The model under review builds one solid part; all positions refer to its coordinate system, in mm. A direction names the side the tool comes from. Give positions to 0.01 mm unless a question says otherwise; leave off trailing zeros. Write each loop counter-clockwise with the first axis right and the second up, starting at its lowest first coordinate (ties: lowest second). Pieces come first, ordered by that corner, then holes.
from build123d import *

# Parameters (mm, degrees)
SKETCH_1_W          = 15
SKETCH_1_H          = 15
SKETCH_1_W_2        = 12
SKETCH_1_H_2        = 12
EXTRUDE_2_DEPTH     = 30
SKETCH_2_R          = 1
CUT_EXTRUDE_1_DEPTH = 10
SKETCH_3_R          = 1.5
CUT_EXTRUDE_2_DEPTH = 10
SKETCH_5_R          = 1.5
CUT_EXTRUDE_4_DEPTH = 10


with BuildPart() as part:
    # ｽｹｯﾁ1 → ﾎﾞｽ - 押し出し2 (new body)
    with BuildSketch(Plane.XY):
        with Locations((0.489915859, 0.232626086)):
            Rectangle(SKETCH_1_W, SKETCH_1_H)
        with Locations((0.489915859, 0.232626086)):
            Rectangle(SKETCH_1_W_2, SKETCH_1_H_2, mode=Mode.SUBTRACT)
    extrude(amount=EXTRUDE_2_DEPTH)

    # ｽｹｯﾁ2 → ｶｯﾄ - 押し出し1 (cut)
    with BuildSketch(Plane(origin=(0, 7.732626086, 0), x_dir=(1, 0, 0), z_dir=(0, 1, 0))):
        with Locations((3.689915859, -25.6)):
            Circle(SKETCH_2_R)
        with Locations((3.689915859, -14.8)):
            Circle(SKETCH_2_R)
    extrude(amount=-CUT_EXTRUDE_1_DEPTH, mode=Mode.SUBTRACT)

    # ｽｹｯﾁ3 → ｶｯﾄ - 押し出し2 (cut)
    with BuildSketch(Plane.ZY.offset(7.010084141)):
        with Locations((7.5, 0.232626086)):
            Circle(SKETCH_3_R)
    extrude(amount=-CUT_EXTRUDE_2_DEPTH, mode=Mode.SUBTRACT)

    # ｽｹｯﾁ5 → ｶｯﾄ - 押し出し4 (cut)
    with BuildSketch(Plane.XZ.offset(7.267373914)):
        with Locations((0.489915859, 22.5)):
            Circle(SKETCH_5_R)
    extrude(amount=-CUT_EXTRUDE_4_DEPTH, mode=Mode.SUBTRACT)


solid = part.part
1) Consider section D-D, the plane x = 3. Give the boundary of the cut face in (y, z).
2) To check wall thickness, follow probe 1 along X at (y, z) = (-2.5, 14.75); probe 2 along Y at (x, z) = (5.25, 24.25); probe 3 along Y at (x, z) = (-6.05, 7.5). State the ranges of each line that lie inside material, in increasing order.
3) Consider section C-C, the plane z = 14.8. Give the boundary of the cut face in (x, y), then the cut area to 3 significant figures.
4) Consider section A-A, the plane x = -1.75. Give the boundary of the cut face in (y, z), then the cut area to 3 significant figures.
5) Insertion check: pin 1 (2.5 mm diameter, centred on x = 0.49, z = 22.5, fed in from -Y). The pin has a flat end and moves straight along its axis. Give the tip position at first contact, or say it passes through.
6) Consider section B-B, the plane y = 5.75. Give the boundary of the cut face in (x, z).
7) Tool access review of faces 4 (the cylindrical face through (-6.27, -0.68, 6.31)), 5 (the cylindrical face through (4.15, 6.99, 15.69)), 6 (the flat face through (-5.51, 0, 15)): name each direction out of +Z, -Z, +X, -X, +Y, -Y from which nothing blocks a thin tool from reaching the whole face with its end or side.
8) The part is to be moulded in two halves that separate along Z. For faces 1 (the flat face through (-6, 0, 0)), 2 (the flat face through (0, -7.267, 15)), 3 (the cylindrical face through (3.56, 6.99, 24.61)), say which applies: +Z half, -Z half, draft (parallel to the pull), parting line (faces both ways), or undercut.
Answer block:
1. outline: (-7.27, 0) - (-5.77, 0) - (-5.77, 30) - (-7.27, 30) - close; (6.23, 0) - (7.73, 0) - (7.73, 14.08) - (6.23, 14.08) - close; (6.23, 15.52) - (7.73, 15.52) - (7.73, 24.88) - (6.23, 24.88) - close; (6.23, 26.32) - (7.73, 26.32) - (7.73, 30) - (6.23, 30) - close
2. probe 1: x = -7.01 to -5.51, 6.49 to 7.99
2. probe 2: y = -7.27 to -5.77, 6.23 to 7.73
2. probe 3: y = -7.27 to -1.27, 1.73 to 7.73
3. outline: (-7.01, -7.27) - (7.99, -7.27) - (7.99, 7.73) - (4.69, 7.73) - (4.69, 6.23) - (6.49, 6.23) - (6.49, -5.77) - (-5.51, -5.77) - (-5.51, 6.23) - (2.69, 6.23) - (2.69, 7.73) - (-7.01, 7.73) - close
3. area: 78.0 mm2
4. outline: (-7.27, 0) - (-5.77, 0) - (-5.77, 30) - (-7.27, 30) - close; (6.23, 0) - (7.73, 0) - (7.73, 30) - (6.23, 30) - close
4. area: 90.0 mm2
5. pin 1: stops at y = 6.23
6. outline: (-7.01, 0) - (-5.51, 0) - (-5.51, 30) - (-7.01, 30) - close; (6.49, 0) - (7.99, 0) - (7.99, 30) - (6.49, 30) - close
7. face 4: -X
7. face 5: +Y
7. face 6: +Z, -Z
8. face 1: -Z half
8. face 2: draft
8. face 3: undercut
